The figure shows three views and two pictorial views of one solid part (mm, origin at its lowest corner). Answer the questions. A direction names the side the tool comes from. Coordinates: 2 decimals unless noted, no trailing zeros. Loops run counter-clockwise (first coordinate to the right, second up) from the corner with the lowest first, then second, coordinate; pieces in that order, holes last.
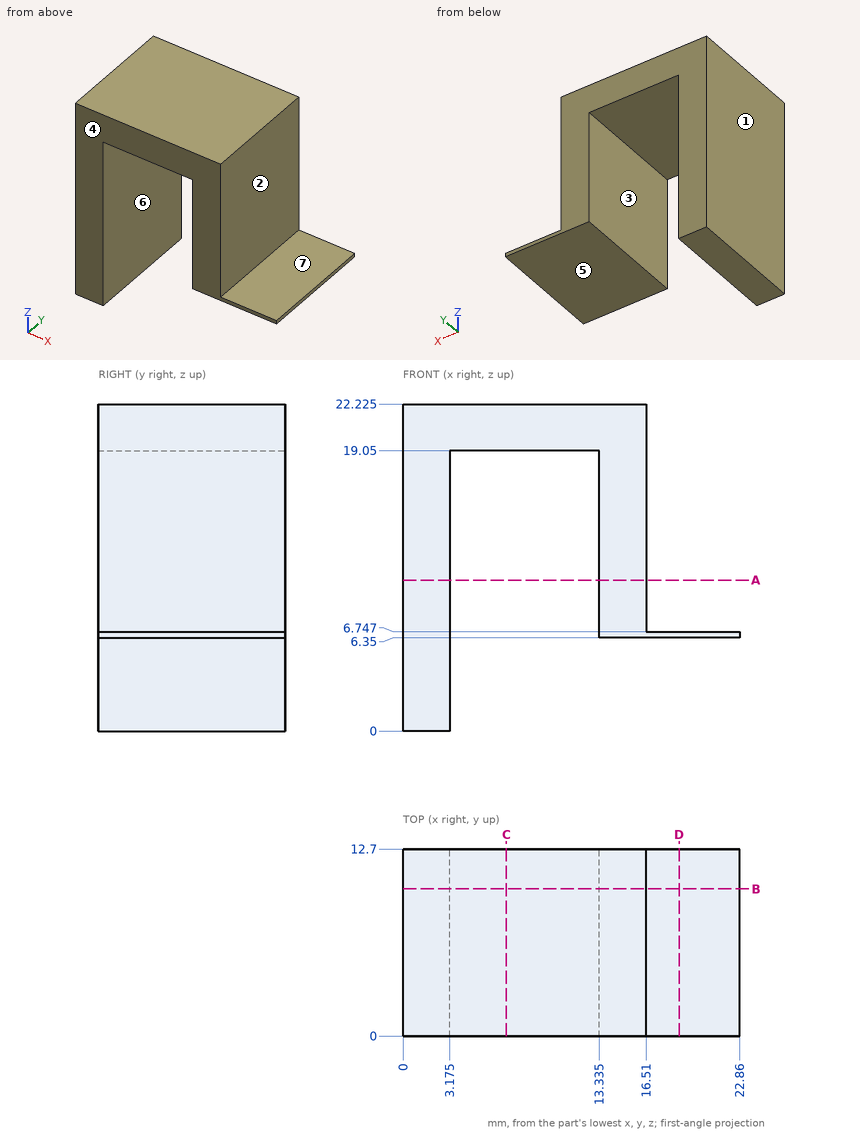
1. A cutting plane is placed at B-B, the plane y = 10. Give the vertices of the cut face in (x, z) (3 decimals).
2. Each of these flat-tipped pins is pushed along its axis until it touches: P1, Ø3, axis at y = 6.5, z = 11.5, coming from the +X side; P2, Ø1.5, axis at x = 20, y = 6, coming from the +Z side; P3, Ø5, axis at x = 20, y = 7, coming from the -Z side. Where does it stop, or does it pass through?
3. Determine the mould class of the marked faces 1, 2, 3 and 4 for opening direction X: released by +X, released by -X, zero draft, split by the parting line, or undercut.
4. Straight lines are drawn through the part: probe 1 along X at (y, z) = (10, 16.25) (3 decimals); probe 2 along Z at (x, y) = (14.25, 10) (3 decimals); probe 3 along Z at (x, y) = (8, 4.75) (3 decimals). For each, find the intervals that lie inside material, in ascending order.
5. A cutting plane is placed at D-D, the plane x = 18.75. Give the vertices of the cut face in (y, z).
6. A cutting plane is placed at C-C, the plane x = 7. Give the vertices of the cut face in (y, z) (3 decimals), then the cut area to 3 significant figures.
7. A cutting plane is placed at A-A, the plane z = 10.25. Give the vertices of the cut face in (x, y) (3 decimals).
8. For the marked faces 5, 6 and 7, determine the directions among +Z, -Z, +X, -X, +Y, -Y from which every point of the face is accessible in a straight line to the end or side of a thin tool.
Answers below:
1. outline: (0, 0) - (3.175, 0) - (3.175, 19.05) - (13.335, 19.05) - (13.335, 6.35) - (22.86, 6.35) - (22.86, 6.747) - (16.51, 6.747) - (16.51, 22.225) - (0, 22.225) - close
2. P1: stops at x = 16.51
2. P2: stops at z = 6.75
2. P3: stops at z = 6.35
3. face 1: released by -X
3. face 2: released by +X
3. face 3: undercut
3. face 4: zero draft
4. probe 1: x = 0 to 3.175, 13.335 to 16.51
4. probe 2: z = 6.35 to 22.225
4. probe 3: z = 19.05 to 22.225
5. outline: (0, 6.35) - (12.7, 6.35) - (12.7, 6.75) - (0, 6.75) - close
6. outline: (0, 19.05) - (12.7, 19.05) - (12.7, 22.225) - (0, 22.225) - close
6. area: 40.3 mm2
7. outline: (0, 0) - (3.175, 0) - (3.175, 12.7) - (0, 12.7) - close; (13.335, 0) - (16.51, 0) - (16.51, 12.7) - (13.335, 12.7) - close
8. face 5: -Z, +X, +Y, -Y
8. face 6: -Z, +Y, -Y
8. face 7: +Z, +X, +Y, -Y
